Could you check a few things on this drawing? It's one solid part, dimensions in mm from its lowest x, y, z. Give positions to 0.01 mm unless a question says otherwise; leave off trailing zeros. Order: outer loops, then holes, each group sorted by start corner. A loop starts at its lowest first (then second) coordinate and runs counter-clockwise, first axis right, second up. Notation, with made-up numbers: (87.5, -17.75) -> (99.5, -17.75) arc R6 ccw to (99.5, -8.75) -> close; hole circle Ø2 at (-19, -21.75). An arc over 180 degrees is marked (long way). Write each question's results on one line, items separated by ' | '. Start each with the question number.
Q1. I need wall thicknesses on line 1 along Y through (x, z) = (5, 39.25); line 2 along X through (y, z) = (6.25, 37) (1 decimal); line 3 along X through (y, z) = (9.5, 9.5). Which ranges of each line are inside material? Lowest first, please. Write a range as [from, to].
Q2. Imagine slicing it at C-C, the plane x = 8.5. Please give me the cut outline in (y, z).
Q3. Imagine slicing it at B-B, the plane x = 2.25. Please give me the cut outline in (y, z) (1 decimal).
Q4. I'm going to push a flat-ended pin straight in: pin 1 (1 mm diameter, centred on x = 1.5, z = 35, fed in from +Y). Where does the tip first touch, or does it pass through?
Q5. Imagine slicing it at A-A, the plane z = 7. Please give me the cut outline in (x, y).
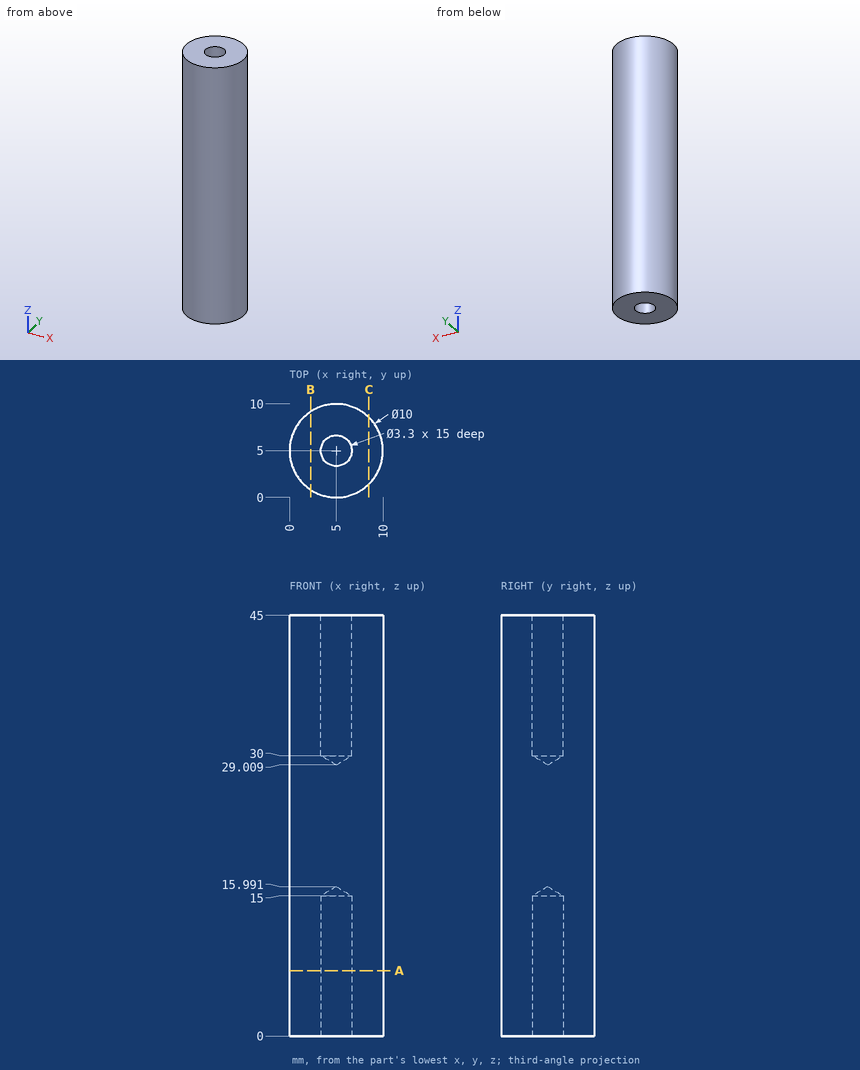
Geometry check:
1) line 1: [0, 3.35], [6.65, 10] | line 2: [0.2, 3.9], [6.1, 9.8] | line 3: [2.82, 7.18]
2) outline: (1.43, 0) -> (8.57, 0) -> (8.57, 45) -> (1.43, 45) -> close
3) outline: (0.8, 0) -> (9.2, 0) -> (9.2, 45) -> (0.8, 45) -> close
4) pin 1: y = 9
5) outline: circle Ø10 at (5, 5); hole circle Ø3.3 at (5, 5)
